Design review of the part built by this model. Coordinates are the model's own, in mm. Round coordinates to 2 decimals unless told otherwise and drop trailing zeros. Loops run counter-clockwise (first coordinate to the right, second up) from the corner with the lowest first, then second, coordinate; pieces in that order, holes last. Notation, with made-up numbers: (66, -16) - (99, -16) arc R28 ccw to (99, 10) - close; hole circle Ø4 at (87.25, 27.5). An arc over 180 degrees is marked (long way). Answer as CSV lines item,"result". Start each with the question number.
(1) Consider section D-D (x = -46). Give the boundary of the cut face in (y, z), and give its area (3 significant figures).
(2) Consider section B-B (y = -83). Give the boundary of the cut face in (x, z).
(3) For P1, Ø1, axis at x = 9, z = -0.5, coming from the +Y side; P2, Ø1.6, axis at x = -15.5, z = 0, coming from the +Y side; P3, Ø1.6, axis at y = -53.5, z = 0, coming from the -X side, all flat-tipped, find the tip position at first contact; note any pin that passes through.
(4) Consider section A-A (z = -0.85). Give the boundary of the cut face in (x, y).
(5) Wall thickness on L1, parallel to Y at x = 0, z = 0.4; L2, parallel to Y at x = -5.5, z = 0.05; L3, parallel to Y at x = 1.5, z = 0.45: over which ranges is each line inside the solid? List them lowest first.
(6) Consider section C-C (y = 0). Give the boundary of the cut face in (x, z).
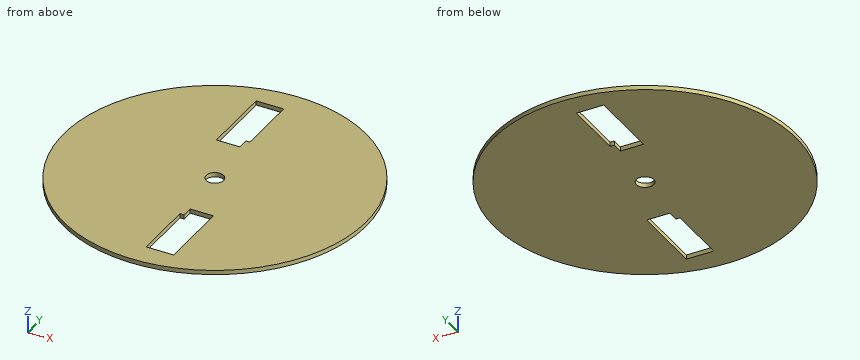
from build123d import *

# Parameters (mm, degrees)
SKETCH1_R           = 110
SKETCH1_R_2         = 6.35
BOSS_EXTRUDE1_DEPTH = 1.5875


with BuildPart() as part:
    # Sketch1 → Boss-Extrude1 (new body, symmetric)
    with BuildSketch(Plane.XY):
        Circle(SKETCH1_R)
        Circle(SKETCH1_R_2, mode=Mode.SUBTRACT)
        Polygon((-6.35, 40), (-3.85, 40), (-3.85, 48), (-0.85, 48), (-0.85, 93), (-20.85, 93), (-20.85, 40), (-18.35, 40), align=None, mode=Mode.SUBTRACT)
        Polygon((6.35, -40), (3.85, -40), (3.85, -48), (0.85, -48), (0.85, -93), (20.85, -93), (20.85, -40), (18.35, -40), align=None, mode=Mode.SUBTRACT)
    extrude(amount=BOSS_EXTRUDE1_DEPTH, both=True)


solid = part.part
Determined:
1,outline,"(-99.92, -1.59) - (99.92, -1.59) - (99.92, 1.59) - (-99.92, 1.59) - close"
1,area,"634 mm^2"
2,outline,"(-72.19, -1.59) - (0.85, -1.59) - (0.85, 1.59) - (-72.19, 1.59) - close; (20.85, -1.59) - (72.19, -1.59) - (72.19, 1.59) - (20.85, 1.59) - close"
3,P1,"stops at y = 109.67"
3,P2,"stops at y = 109.01"
3,P3,"stops at x = -96.55"
4,outline,"circle Ø220 at (0, 0); hole (-20.85, 40) - (-3.85, 40) - (-3.85, 48) - (-0.85, 48) - (-0.85, 93) - (-20.85, 93) - close; hole circle Ø12.7 at (0, 0); hole (0.85, -93) - (20.85, -93) - (20.85, -40) - (3.85, -40) - (3.85, -48) - (0.85, -48) - close"
5,L1,"y = -110 to -6.35, 6.35 to 110"
5,L2,"y = -109.86 to -3.17, 3.17 to 40, 93 to 109.86"
5,L3,"y = -109.99 to -93, -48 to -6.17, 6.17 to 109.99"
6,outline,"(-110, -1.59) - (-6.35, -1.59) - (-6.35, 1.59) - (-110, 1.59) - close; (6.35, -1.59) - (110, -1.59) - (110, 1.59) - (6.35, 1.59) - close"
